```python
from build123d import *

# Parameters (mm, degrees)
SKETCH2_W           = 398.100558659
SKETCH2_H           = 70
BOSS_EXTRUDE1_DEPTH = 20
CUT_EXTRUDE1_DEPTH  = 10
SKETCH4_R           = 2.921
BOSS_EXTRUDE2_DEPTH = 10


with BuildPart() as part:
    # Sketch2 → Boss-Extrude1 (new body)
    with BuildSketch(Plane(origin=(0, 0, 0), x_dir=(0, 0, -1), z_dir=(1, 0, 0))):
        with Locations((199.05027933, 35)):
            Rectangle(SKETCH2_W, SKETCH2_H)
    extrude(amount=BOSS_EXTRUDE1_DEPTH)

    # Sketch3 → Cut-Extrude1 (cut)
    with BuildSketch(Plane(origin=(20, 0, 0), x_dir=(0, 0, -1), z_dir=(1, 0, 0))):
        with BuildLine():
            Line((35, 52.5), (363.100558659, 52.5))
            ThreePointArc((363.100558659, 52.5), (380.600558659, 35), (363.100558659, 17.5))
            Line((363.100558659, 17.5), (35, 17.5))
            ThreePointArc((35, 17.5), (17.5, 35), (35, 52.5))
        make_face()
    extrude(amount=-CUT_EXTRUDE1_DEPTH, mode=Mode.SUBTRACT)

    # Sketch4 → Boss-Extrude2 (add)
    with BuildSketch(Plane.ZY):
        with Locations((-391.750558659, 35)):
            Circle(SKETCH4_R)
        with Locations(Location((-6.35, 35, 0), (0, 0, 180))):
            Circle(SKETCH4_R)
    extrude(amount=BOSS_EXTRUDE2_DEPTH)


solid = part.part
```
Could you check a few things on this model? Use its own coordinates, in mm. A direction names the side the tool comes from. Give positions to 0.01 mm unless a question says otherwise; leave off trailing zeros. Order: outer loops, then holes, each group sorted by start corner. A loop starts at its lowest first (then second) coordinate and runs counter-clockwise, first axis right, second up.
Q1. Suppose I cut it at C-C, the plane y = 10. Write out the boundary of the cut face in (x, z), and give its area (3 significant figures).
Q2. For faces 1 (the cylindrical face through (15.07, 34.615, -17.504)), 2 (the flat face through (10, 35, -398.101)), which set-ups out of +Z, -Z, +X, -X, +Y, -Y let a thin tool reach every point of the face, with its end or its side?
Q3. We'd pull the mould along Y, two halves only. Please class faces 3 (the flat face through (10, 0, -196)), 4 (the flat face through (10, 35, 0)), 5 (the cylindrical face through (15.07, 35.385, -380.596)): +Y half, -Y half, draft (parallel to the pull), parting line (faces both ways), or undercut.
Q4. Suppose I cut it at A-A, the plane z = -279. Write out the boundary of the cut face in (x, y), and give its area (3 significant figures).
Q5. Suppose I cut it at B-B, the plane y = 24.5. Write out the boundary of the cut face in (x, z), and give its area (3 significant figures).
Q6. I'm going to push flat-ended pins straight in: P1, Ø12, axis at y = 41.5, z = -341.5, coming from the -X side; P2, Ø6, axis at x = -4, z = -168.5, coming from the -Y side. Where does each tip first touch, or does it pass through?
Q7. If I drill on line 1 along Y through (x, z) = (10.5, -99); line 2 along X through (y, z) = (29, -160); line 3 along X through (y, z) = (67.5, -88), over which ranges is the centre line in solid material (lowest first)?
Solution:
1. outline: (0, -398.1) - (20, -398.1) - (20, 0) - (0, 0) - close
1. area: 7,960 mm2
2. face 1: +X
2. face 2: -Z, +X, -X, +Y, -Y
3. face 3: -Y half
3. face 4: draft
3. face 5: undercut
4. outline: (0, 0) - (20, 0) - (20, 17.5) - (10, 17.5) - (10, 52.5) - (20, 52.5) - (20, 70) - (0, 70) - close
4. area: 1,050 mm2
5. outline: (0, -398.1) - (20, -398.1) - (20, -377.1) - (10, -377.1) - (10, -21) - (20, -21) - (20, 0) - (0, 0) - close
5. area: 4,400 mm2
6. P1: stops at x = 0
6. P2: passes through
7. line 1: y = 0 to 17.5, 52.5 to 70
7. line 2: x = 0 to 10
7. line 3: x = 0 to 20
